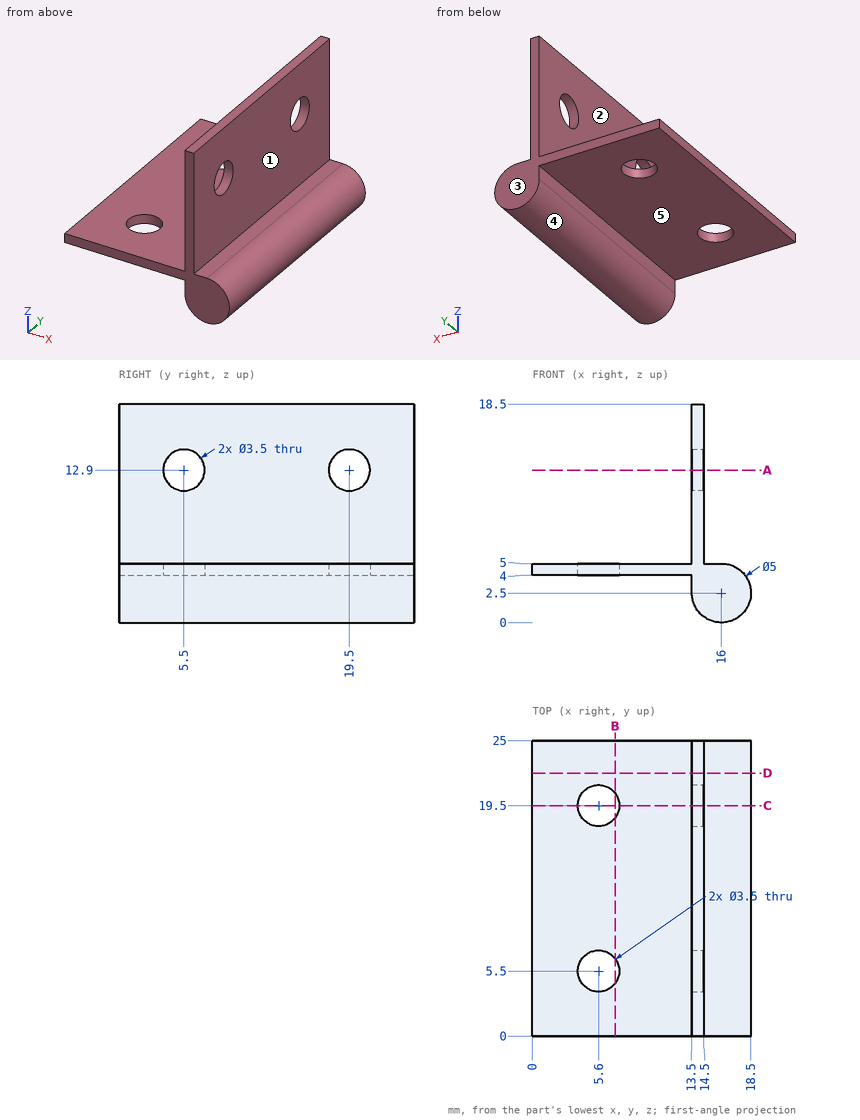
Design review of the part shown in the three views and the two pictorial views. Dimensions are in mm from the part's minimum x, y and z. A direction names the side the tool comes from. Round coordinates to 2 decimals unless told otherwise and drop trailing zeros. Write each loop counter-clockwise with the first axis right and the second up, starting at its lowest first coordinate (ties: lowest second). Pieces come first, ordered by that corner, then holes. Notation, with made-up numbers: (26, -16.5) - (79, -16.5) arc R5 ccw to (79, -10.5) - close; hole circle Ø10 at (23, -36). An arc over 180 degrees is marked (long way). Return JSON: item names as keys, results as strings. Group by question number.
Item 1: Insertion check: P1, Ø5, axis at y = 18.5, z = 14.5, coming from the -X side; P2, Ø4, axis at x = 2.5, y = 13.5, coming from the -Z side; P3, Ø4, axis at y = 5.5, z = 12.9, coming from the +X side. Each pin has a flat end and moves straight along its axis. Give the tip position at first contact, or say it passes through.
Item 2: Machinability: for the marked faces 1, 2, 3, 4 and 5, which of the approach directions +Z, -Z, +X, -X, +Y, -Y give a long, thin tool a straight path to every point of the face, cutting with its end or side? Answer none if there is none.
Item 3: We need section A-A on z = 12.9. Write out the cut boundary in (x, y).
Item 4: We need section D-D on y = 22.25. Write out the cut boundary in (x, z).
Item 5: We need section B-B on x = 7. Write out the cut boundary in (y, z), and give its area (3 significant figures).
Item 6: We need section C-C on y = 19.5. Write out the cut boundary in (x, z), and give its area (3 significant figures).
Item 7: For probe 1 along Y at (x, z) = (5.6, 4.5); probe 2 along Z at (x, y) = (6.25, 14.75); probe 3 along X at (y, z) = (12.25, 7.25), list the stretches that pass through material, from the lowest coordinate up. Write a range as [from, to].
Model answer:
{
 "1": {"P1": "stops at x = 13.5", "P2": "stops at z = 4", "P3": "stops at x = 14.5"},
 "2": {"face 1": "+Z, +X, +Y, -Y", "face 2": "+Z, -X, +Y, -Y", "face 3": "+Z, -Z, +X, -X, +Y", "face 4": "+Y, -Y", "face 5": "-Z, -X, +Y, -Y"},
 "3": {"outline": "(13.5, 0) - (14.5, 0) - (14.5, 3.75) - (13.5, 3.75) - close; (13.5, 7.25) - (14.5, 7.25) - (14.5, 17.75) - (13.5, 17.75) - close; (13.5, 21.25) - (14.5, 21.25) - (14.5, 25) - (13.5, 25) - close"},
 "4": {"outline": "(0, 4) - (13.5, 4) - (13.5, 2.5) arc R2.5 ccw (long way) to (16, 5) - (14.5, 5) - (14.5, 18.5) - (13.5, 18.5) - (13.5, 5) - (0, 5) - close"},
 "5": {"outline": "(0, 4) - (4.45, 4) - (4.45, 5) - (0, 5) - close; (6.55, 4) - (18.45, 4) - (18.45, 5) - (6.55, 5) - close; (20.55, 4) - (25, 4) - (25, 5) - (20.55, 5) - close", "area": "20.8 mm²"},
 "6": {"outline": "(0, 4) - (3.85, 4) - (3.85, 5) - (0, 5) - close; (7.35, 4) - (13.5, 4) - (13.5, 2.5) arc R2.5 ccw (long way) to (16, 5) - (14.5, 5) - (14.5, 11.15) - (13.5, 11.15) - (13.5, 5) - (7.35, 5) - close; (13.5, 14.65) - (14.5, 14.65) - (14.5, 18.5) - (13.5, 18.5) - close", "area": "41.0 mm²"},
 "7": {"probe 1": "y = [0, 3.75], [7.25, 17.75], [21.25, 25]", "probe 2": "z = [4, 5]", "probe 3": "x = [13.5, 14.5]"}
}
